Autodesk Inventor part; units mm, degrees
ref_plane "YZ Plane" through (0, 0, 0) normal (1, 0, 0) x (0, 1, 0)
ref_plane "XZ Plane" through (0, 0, 0) normal (0, 1, 0) x (-1, 0, 0)
ref_plane "XY Plane" through (0, 0, 0) normal (0, 0, 1) x (1, 0, 0)
sketch "Sketch1" plane through (0, 0, 0) normal (0, 1, 0) x (-1, 0, 0)
  circle A0 centre (0, 0) radius 10
  dimension "d0" = 20
extrude "Extrusion1" add sketch "Sketch1" along normal blind 15
sketch "Sketch2" plane through (0, 15, 0) normal (0, 1, 0) x (1, 0, 0)
  circle A0 centre (0, 0) radius 4
  circle A1 centre (0, 0) radius 8
  circle A2 centre (0, 0) radius 10
  dimension "d3" = 8
  dimension "d4" = 2
extrude "Extrusion2" cut sketch "Sketch2" against normal blind 9 contours A1
sketch "Sketch3" plane through (0, 6, 0) normal (0, 1, 0) x (1, 0, 0)
  circle A0 centre (0, 0) radius 4
  circle A1 centre (0, 0) radius 4
  circle A2 centre (0, 0) radius 8
  circle A3 centre (0, 0) radius 8
extrude "Extrusion3" add sketch "Sketch3" along normal blind 8
sketch "Sketch5" plane through (0, 15, 0) normal (0, 1, 0) x (1, 0, 0)
  circle A0 centre (0, 0) radius 4
  circle A1 centre (0, 0) radius 2
  dimension "d20" = 4
hole "Hole2" at (0, 15, 0) direction (0, -1, 0) diameter 3.242 end through all countersink diameter 6 countersink angle 90
properties part number "20-15 Electromagnet"
Can you work these out from the model? Positions are in its coordinate system, mm. A direction names the side the tool comes from. Coordinates: 2 decimals unless noted, no trailing zeros. Loops run counter-clockwise (first coordinate to the right, second up) from the corner with the lowest first, then second, coordinate; pieces in that order, holes last. Notation, with made-up numbers: (-19.75, 19.25) -> (25.25, 19.25) arc R20 cw to (25.25, 43.25) -> close; hole circle Ø8 at (-27, 72). An arc over 180 degrees is marked (long way). Put each result on its own line as item: value. Start each with the question number.
Q1. I want a section at B-B (z = 0). Write out the boundary of the cut face in (x, y).
Q2. I want a section at C-C (y = 4.25). Write out the boundary of the cut face in (x, z), plus the area to 3 significant figures.
Q3. If I drill on line 1 (Z direction, x = 0, y = 14.45); line 2 (Z direction, x = 0, y = 14.3); line 3 (Z direction, x = -6, y = 10.75), over which ranges is the centre line in solid material (lowest first)? Write a range as [from, to].
Q4. I want a section at D-D (x = 7.5). Write out the boundary of the cut face in (y, z), plus the area to 3 significant figures.
Q5. Thinking about a two-plate mould opening in X: for faces 3 (the face through (-0.867, 14.507, 3.905)), 4 (the face through (2.17, 7.4, 9.76)), 5 (the face through (0, 15, 8.2)), which applies, pulls with the +X half, pulls with the -X half, needs draft (parallel to the pull), parting line crosses it, or undercut?
Q6. I'm going to push flat-ended pins straight in: P1, Ø1.5, axis at x = -1.5, y = 8, coming from the -Z side; P2, Ø2, axis at y = 2.5, z = -2, coming from the +X side; P3, Ø5, axis at x = 4, y = 13, coming from the -Z side. Where does each tip first touch, or does it pass through?
Q7. I want a section at A-A (x = 0). Write out the boundary of the cut face in (y, z).
Q8. For faces 1 (the face through (-1.73, 14.51, 7.81)), 2 (the face through (1.438, 6.715, 0.748)), which set-ups out of +Z, -Z, +X, -X, +Y, -Y let a thin tool reach every point of the face, with its end or its side?
Taken from the geometry:
1. outline: (-10, 0) -> (-1.62, 0) -> (-1.62, 13.62) -> (-3, 15) -> (-4, 15) -> (-4, 14) -> (-8, 14) -> (-8, 15) -> (-10, 15) -> close; (1.62, 0) -> (10, 0) -> (10, 15) -> (8, 15) -> (8, 14) -> (4, 14) -> (4, 15) -> (3, 15) -> (1.62, 13.62) -> close
2. outline: circle Ø20 at (0, 0); hole circle Ø3.24 at (0, 0)
2. area: 306 mm2
3. line 1: z = [-10, -8], [-4, -2.45], [2.45, 4], [8, 10]
3. line 2: z = [-10, -8], [-4, -2.3], [2.3, 4], [8, 10]
3. line 3: z = [-8, 8]
4. outline: (0, -6.61) -> (15, -6.61) -> (15, -2.78) -> (14, -2.78) -> (14, 2.78) -> (15, 2.78) -> (15, 6.61) -> (0, 6.61) -> close
4. area: 193 mm2
5. face 3: undercut
5. face 4: parting line crosses it
5. face 5: needs draft
6. P1: stops at z = -9.97
6. P2: stops at x = 9.95
6. P3: stops at z = -9.89
7. outline: (0, -10) -> (15, -10) -> (15, -8) -> (14, -8) -> (14, -4) -> (15, -4) -> (15, -3) -> (13.62, -1.62) -> (0, -1.62) -> close; (0, 1.62) -> (13.62, 1.62) -> (15, 3) -> (15, 4) -> (14, 4) -> (14, 8) -> (15, 8) -> (15, 10) -> (0, 10) -> close
8. face 1: +Y
8. face 2: +Y, -Y
